Input: part model. Units: mm. Frame: model coordinates. A direction names the side the tool comes from. Round coordinates to 2 decimals unless told otherwise and drop trailing zeros. Write each loop counter-clockwise with the first axis right and the second up, starting at its lowest first coordinate (ties: lowest second). Pieces come first, ordered by that corner, then holes. Notation, with made-up numbers: (-38.75, 84.25) -> (-29.75, 84.25) arc R16 cw to (-29.75, 103.25) -> close; hole circle Ø4 at (28.25, -8). An arc over 180 degrees is marked (long way). Write item = value, one per line. Start each with the question number.
```python
from build123d import *

# Parameters (mm, degrees)
EXTRUDE_1_DEPTH      = 30
SKETCH_2_R           = 1.5
CUT_EXTRUDE_1_DEPTH  = 5
CUT_EXTRUDE_4_DEPTH  = 307
SKETCH_3_W           = 285.26
SKETCH_3_H           = 138.01
CUT_EXTRUDE_5_DEPTH  = 13
SKETCH_12_W          = 40
SKETCH_12_H          = 50
CUT_EXTRUDE_7_DEPTH  = 3
CUT_EXTRUDE_7_DRAFT  = -30
SKETCH_9_W           = 100
SKETCH_9_H           = 80
CUT_EXTRUDE_8_DEPTH  = 3
CUT_EXTRUDE_8_DRAFT  = -30
CUT_EXTRUDE_9_DEPTH  = 11
FILLET_1_R           = 2
CUT_EXTRUDE_10_DEPTH = 11
FILLET_2_R           = 2
FILLET_3_R           = 2
FILLET_4_R           = 2
EXTRUDE_3_DEPTH      = 5
EXTRUDE_4_DEPTH      = 5


with BuildPart() as part:
    # Model → 凸台-拉伸1 (new body)
    with BuildSketch(Plane.XY):
        with BuildLine():
            Line((0, 11), (0, 150.75))
            ThreePointArc((0, 150.75), (2.343145751, 156.406854249), (8, 158.75))
            Line((8, 158.75), (298.011203897, 158.75))
            ThreePointArc((298.011203897, 158.75), (303.664092807, 156.410816811), (306.011196041, 150.761211743))
            Line((306.011196041, 150.761211743), (306.207051361, 11.011211743))
            Line((306.207051361, 11.011211743), (306.207051361, 8))
            ThreePointArc((306.207051361, 8), (303.863905611, 2.343145751), (298.207051361, 0))
            Line((298.207051361, 0), (8, 0))
            ThreePointArc((8, 0), (2.343145751, 2.343145751), (0, 8))
            Line((0, 8), (0, 11))
        make_face()
    extrude(amount=-EXTRUDE_1_DEPTH)

    # 草图2 → 切除-拉伸1 (cut)
    with BuildSketch(Plane.XY):
        with Locations((105.108569936, 3.75)):
            Circle(SKETCH_2_R)
        with Locations((9.108569936, 3.75)):
            Circle(SKETCH_2_R)
        with Locations((201.10846029, 3.817270412)):
            Circle(SKETCH_2_R)
        with Locations((297.108366012, 3.951811323)):
            Circle(SKETCH_2_R)
        with Locations((105.108569936, 155)):
            Circle(SKETCH_2_R)
        with Locations((9.108569936, 155)):
            Circle(SKETCH_2_R)
        with Locations((201.10846029, 154.932729588)):
            Circle(SKETCH_2_R)
        with Locations((297.108366012, 154.798188677)):
            Circle(SKETCH_2_R)
        with Locations((3.75, 109.375)):
            Circle(SKETCH_2_R)
        with Locations((3.75, 49.375)):
            Circle(SKETCH_2_R)
        with Locations((302.318900647, 109.584217456)):
            Circle(SKETCH_2_R)
        with Locations((302.402988717, 49.58427638)):
            Circle(SKETCH_2_R)
    extrude(amount=-CUT_EXTRUDE_1_DEPTH, mode=Mode.SUBTRACT)

    # 草图6 → 切除-拉伸4 (cut)
    with BuildSketch(Plane.ZY):
        Polygon((-30, 158.75), (-30, 0), (-15, 0), align=None)
    extrude(amount=-CUT_EXTRUDE_4_DEPTH, mode=Mode.SUBTRACT)

    # 草图3 → 切除-拉伸5 (cut)
    with BuildSketch(Plane.XY):
        with Locations((153, 79.375)):
            Rectangle(SKETCH_3_W, SKETCH_3_H)
    extrude(amount=-CUT_EXTRUDE_5_DEPTH, mode=Mode.SUBTRACT)


with BuildPart() as cut_extrude_7_tool:
    # 草图12 → 切除-拉伸7 (with draft: the straight prism first)
    with BuildSketch(Plane.XY.offset(-13)):
        with Locations((153, 70.37)):
            Rectangle(SKETCH_12_W, SKETCH_12_H)
    extrude(amount=-CUT_EXTRUDE_7_DEPTH)
    # 切除-拉伸7: the draft: its side faces are tilted about the plane it starts from
    cut_extrude_7_sides = [cut_extrude_7_tool.faces().sort_by_distance(p)[0] for p in [
        (153, 45.37, -14.5),
        (173, 70.37, -14.5),
        (153, 95.37, -14.5),
        (133, 70.37, -14.5),
    ]]
    draft(cut_extrude_7_sides, Plane.XY.offset(-13), CUT_EXTRUDE_7_DRAFT)


with BuildPart() as part_1:
    add(part.part)

    # 切除-拉伸7: cut by cut_extrude_7_tool
    add(cut_extrude_7_tool.part, mode=Mode.SUBTRACT)


with BuildPart() as cut_extrude_8_tool:
    # 草图9 → 切除-拉伸8 (with draft: the straight prism first)
    with BuildSketch(Plane.XY.offset(-13)):
        with Locations((75.37, 88.38)):
            Rectangle(SKETCH_9_W, SKETCH_9_H)
    extrude(amount=-CUT_EXTRUDE_8_DEPTH)
    # 切除-拉伸8: the draft: its side faces are tilted about the plane it starts from
    cut_extrude_8_sides = [cut_extrude_8_tool.faces().sort_by_distance(p)[0] for p in [
        (25.37, 88.38, -14.5),
        (75.37, 48.38, -14.5),
        (125.37, 88.38, -14.5),
        (75.37, 128.38, -14.5),
    ]]
    draft(cut_extrude_8_sides, Plane.XY.offset(-13), CUT_EXTRUDE_8_DRAFT)


with BuildPart() as part_2:
    add(part_1.part)

    # 切除-拉伸8: cut by cut_extrude_8_tool
    add(cut_extrude_8_tool.part, mode=Mode.SUBTRACT)

    # 草图14 → 切除-拉伸9 (cut)
    with BuildSketch(Plane.ZY):
        with BuildLine():
            Line((-5.9, 129.38), (-6.1, 129.38))
            ThreePointArc((-6.1, 129.38), (-7.797056275, 128.677056275), (-8.5, 126.98))
            Line((-8.5, 126.98), (-8.5, 120.78))
            ThreePointArc((-8.5, 120.78), (-7.797056275, 119.082943725), (-6.1, 118.38))
            Line((-6.1, 118.38), (-5.9, 118.38))
            ThreePointArc((-5.9, 118.38), (-4.202943725, 119.082943725), (-3.5, 120.78))
            Line((-3.5, 120.78), (-3.5, 126.98))
            ThreePointArc((-3.5, 126.98), (-4.202943725, 128.677056275), (-5.9, 129.38))
        make_face()
    extrude(amount=-CUT_EXTRUDE_9_DEPTH, mode=Mode.SUBTRACT)

    # 圆角1
    fillet_1_edges = [part_2.edges().sort_by_distance(p)[0] for p in [
        (0, 123.88, -3.5),
        (0, 118.38, -6),
        (0, 119.082943725, -7.797056275),
        (0, 128.677056275, -7.797056275),
        (0, 128.677056275, -4.202943725),
        (0, 129.38, -6),
        (0, 123.88, -8.5),
        (0, 119.082943725, -4.202943725),
    ]]
    fillet(fillet_1_edges, radius=FILLET_1_R)

    # 草图15 → 切除-拉伸10 (cut)
    with BuildSketch(Plane.XZ):
        with BuildLine():
            Line((222.53, -3.959687417), (229.73, -3.959687417))
            ThreePointArc((229.73, -3.959687417), (231.427056275, -4.662631142), (232.13, -6.359687417))
            Line((232.13, -6.359687417), (232.13, -6.559687417))
            ThreePointArc((232.13, -6.559687417), (231.427056275, -8.256743692), (229.73, -8.959687417))
            Line((229.73, -8.959687417), (222.53, -8.959687417))
            ThreePointArc((222.53, -8.959687417), (220.832943725, -8.256743692), (220.13, -6.559687417))
            Line((220.13, -6.559687417), (220.13, -6.359687417))
            ThreePointArc((220.13, -6.359687417), (220.832943725, -4.662631142), (222.53, -3.959687417))
        make_face()
    extrude(amount=-CUT_EXTRUDE_10_DEPTH, mode=Mode.SUBTRACT)

    # 圆角2
    fillet_2_edges = [part_2.edges().sort_by_distance(p)[0] for p in [
        (226.13, 0, -3.959687417),
        (232.13, 0, -6.459687417),
        (231.427056275, 0, -8.256743692),
        (220.832943725, 0, -4.662631142),
        (220.13, 0, -6.459687417),
        (220.832943725, 0, -8.256743692),
        (226.13, 0, -8.959687417),
        (231.427056275, 0, -4.662631142),
    ]]
    fillet(fillet_2_edges, radius=FILLET_2_R)

    # 圆角3
    fillet_3_edges = [part_2.edges().sort_by_distance(p)[0] for p in [
        (10.37, 129.38, -6),
        (10.37, 128.677056275, -7.797056275),
        (10.37, 123.88, -8.5),
        (10.37, 119.082943725, -7.797056275),
        (10.37, 118.38, -6),
        (10.37, 119.082943725, -4.202943725),
        (10.37, 123.88, -3.5),
        (10.37, 128.677056275, -4.202943725),
    ]]
    fillet(fillet_3_edges, radius=FILLET_3_R)

    # 圆角4
    fillet_4_edges = [part_2.edges().sort_by_distance(p)[0] for p in [
        (220.13, 10.37, -6.459687417),
        (220.832943725, 10.37, -8.256743692),
        (226.13, 10.37, -8.959687417),
        (231.427056275, 10.37, -8.256743692),
        (232.13, 10.37, -6.459687417),
        (231.427056275, 10.37, -4.662631142),
        (226.13, 10.37, -3.959687417),
        (220.832943725, 10.37, -4.662631142),
    ]]
    fillet(fillet_4_edges, radius=FILLET_4_R)


with BuildPart() as body_2:
    # Split Bodies 1: the piece on the far side of the plane
    add(part_2.part)
    split(bisect_by=Plane(origin=(153.005601949, 0, 0), x_dir=(0, 0, 1), z_dir=(1, 0, 0)), keep=Keep.BOTTOM)


with BuildPart() as part_3:
    add(part_2.part)

    # Split Bodies 1
    split(bisect_by=Plane(origin=(153.005601949, 0, 0), x_dir=(0, 0, 1), z_dir=(1, 0, 0)), keep=Keep.TOP)

    # 草图19 → 凸台-拉伸3 (add)
    with BuildSketch(Plane.ZY.offset(-153.005601949)):
        Polygon((-19.286929134, 45.37), (-15, 0), (-13, 0), (-13, 10.37), (-13, 45.37), (-16, 47.102050808), align=None)
    extrude(amount=EXTRUDE_3_DEPTH)

    # 草图19<5> → 凸台-拉伸4 (add)
    with BuildSketch(Plane.ZY.offset(-153.005601949)):
        Polygon((-30, 158.75), (-24.011338583, 95.37), (-16, 93.637949192), (-13, 95.37), (-13, 148.38), (-13, 158.75), align=None)
        Polygon((-19.286929134, 45.37), (-15, 0), (-13, 0), (-13, 10.37), (-13, 45.37), (-16, 47.102050808), align=None)
    extrude(amount=EXTRUDE_4_DEPTH)


solid = part_3.part
```
1. Section A-A (x = 227). Output: boundary loops of the cut face in (y, z), then the cut area to 3 significant figures.
2. Pin query (flat end, axial travel): P1, Ø2.5, axis at x = 296.5, y = 4, coming from the +Z side; P2, Ø2.5, axis at x = 201.11, y = 3.82, coming from the -Z side; P3, Ø12, axis at y = 92, z = -22, coming from the +X side; P4, Ø3.5, axis at x = 302.32, y = 109.58, coming from the -Z side. Return the tip coordinate at first contact, or that it passes through.
3. Reachability of faces 1 (the flat face through (223, 10.37, -12)), 2 (the flat face through (153.006, 5, -7)), 3 (the flat face through (150.541, 94.516, -20.062)) from +Z, -Z, +X, -X, +Y, -Y: full face, straight path, thin tool, end or side. Return the list, or none.
4. Section B-B (x = 187). Output: boundary loops of the cut face in (y, z), then the cut area to 3 significant figures.
5. Section D-D (x = 163). Output: boundary loops of the cut face in (y, z), then the cut area to 3 significant figures.
6. Mould query, pull axis Z, two halves, no side actions, for faces 4 (the flat face through (226, 5, -3.96)), 5 (the flat face through (226, 5, -8.96)), 6 (the flat face through (162, 71, -16)), 7 (the cylindrical face through (303.602, 156.473, -14.79)). Classes: pulls with the +Z half, pulls with the -Z half, needs draft (parallel to the pull), parting line crosses it, or undercut.
7. Section C-C (y = 59). Output: boundary loops of the cut face in (x, z).
8. Line query: line 1 along Y through (x, z) = (190, -4.5); line 2 along Z through (x, y) = (230, 11); line 3 along X through (y, z) = (123, -12). Output: solid intervals per line, ascending.
Check sheet entries:
q1.outline = (0, -15) -> (158.75, -30) -> (158.75, 0) -> (148.38, 0) -> (148.38, -13) -> (10.37, -13) -> (10.37, -10.96) arc R2 ccw to (8.37, -8.96) -> (2, -8.96) arc R2 ccw to (0, -10.96) -> close; (0, -1.96) arc R2 ccw to (2, -3.96) -> (8.37, -3.96) arc R2 ccw to (10.37, -1.96) -> (10.37, 0) -> (0, 0) -> close
q1.area = 1,720 mm2
q2.P1 = 0
q2.P2 = -15.48
q2.P3 = 306.1
q2.P4 = -25.52
q3.face_1 = +Z, -X
q3.face_2 = +Z, -X, +Y, -Y
q3.face_3 = -Z, -X
q4.outline = (0, -15) -> (158.75, -30) -> (158.75, 0) -> (148.38, 0) -> (148.38, -13) -> (10.37, -13) -> (10.37, 0) -> (0, 0) -> close
q4.area = 1,780 mm2
q5.outline = (0, -15) -> (158.75, -30) -> (158.75, 0) -> (148.38, 0) -> (148.38, -13) -> (95.37, -13) -> (93.64, -16) -> (47.1, -16) -> (45.37, -13) -> (10.37, -13) -> (10.37, 0) -> (0, 0) -> close
q5.area = 1,630 mm2
q6.face_4 = undercut
q6.face_5 = undercut
q6.face_6 = pulls with the +Z half
q6.face_7 = needs draft
q7.outline = (153.01, -20.57) -> (306.14, -20.57) -> (306.14, 0) -> (295.63, 0) -> (295.63, -13) -> (173, -13) -> (171.27, -16) -> (153.01, -16) -> close
q8.line_1 = 0 to 10.37, 148.38 to 158.75
q8.line_2 = -16.04 to -13
q8.line_3 = 295.63 to 306.05
